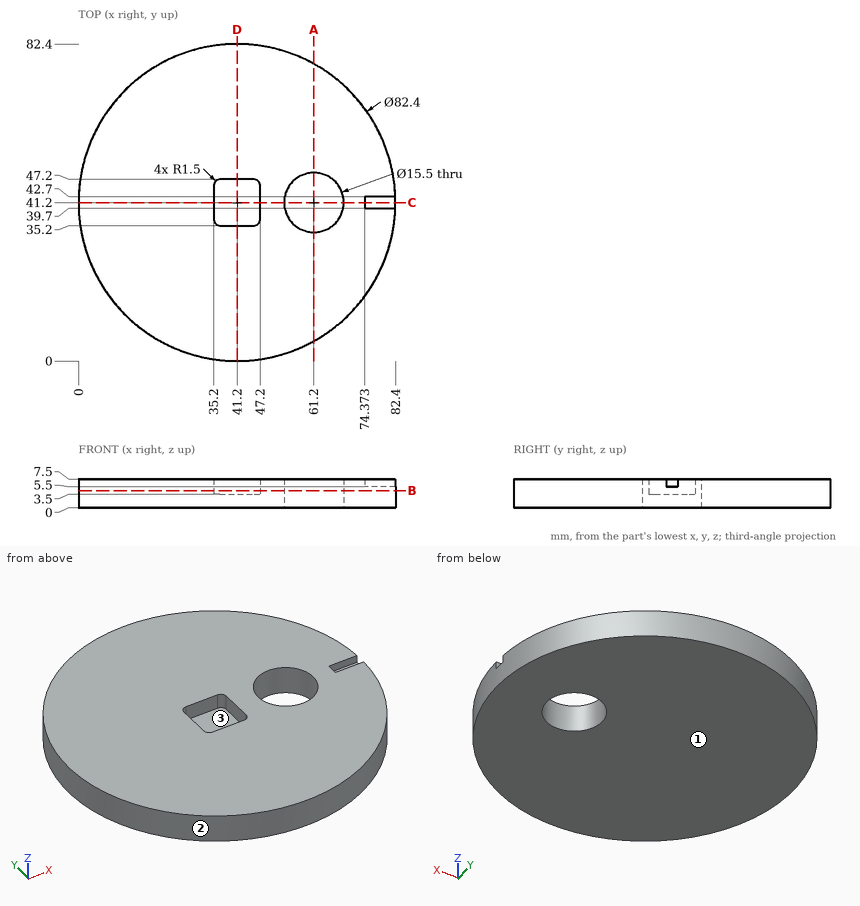
Geometry: see drawing. Coordinates: mm, zero at the bounding-box minimum. Round coordinates to 2 decimals unless told otherwise and drop trailing zeros. Order: outer loops, then holes, each group sorted by start corner. A loop starts at its lowest first (then second) coordinate and runs counter-clockwise, first axis right, second up. Notation, with made-up numbers: (28.5, -22.75) - (57.5, -22.75) arc R19 ccw to (57.5, -2.75) - close; hole circle Ø10 at (23, 33). An arc over 180 degrees is marked (long way). One line per question, with ' | ' between items. Start each with the question number.
1) Cut plane B-B, the plane z = 4.5. Return the cut outline in (x, y).
2) Ray query, probe 1 along X at (y, z) = (41.2, 4.75); probe 2 along X at (y, z) = (41.2, 2); probe 3 along Y at (x, z) = (61.2, 4.5). Return the intervals inside material, ascending.
3) Cut plane C-C, the plane y = 41.2. Return the cut outline in (x, z), then the cut area to 3 significant figures.
4) Cut plane D-D, the plane x = 41.2. Return the cut outline in (y, z).
5) Pull-direction query (X, two-part tool) for the marked faces 1, 2 and 3; classes: +X half, -X half, draft (parallel to the pull), parting line (faces both ways), or undercut.
6) Cut plane A-A, the plane x = 61.2. Return the cut outline in (y, z), then the cut area to 3 significant figures.
7) Contact query for flat-ended pins moving along their axis: P1, Ø4, axis at x = 66, z = 6, coming from the -Y side; P2, Ø0.6, axis at x = 78, z = 6, coming from the +Y side; P3, Ø1.5, axis at x = 44, z = 3, coming from the -Y side. Output: stop coordinate, or through.
Worked out:
1) outline: circle Ø82.4 at (41.2, 41.2); hole (35.2, 36.7) arc R1.5 ccw to (36.7, 35.2) - (45.7, 35.2) arc R1.5 ccw to (47.2, 36.7) - (47.2, 45.7) arc R1.5 ccw to (45.7, 47.2) - (36.7, 47.2) arc R1.5 ccw to (35.2, 45.7) - close; hole circle Ø15.5 at (61.2, 41.2)
2) probe 1: x = 0 to 35.2, 47.2 to 53.45, 68.95 to 82.4 | probe 2: x = 0 to 53.45, 68.95 to 82.4 | probe 3: y = 5.18 to 33.45, 48.95 to 77.22
3) outline: (0, 0) - (53.45, 0) - (53.45, 7.5) - (47.2, 7.5) - (47.2, 3.5) - (35.2, 3.5) - (35.2, 7.5) - (0, 7.5) - close; (68.95, 0) - (82.4, 0) - (82.4, 5.5) - (74.37, 5.5) - (74.37, 7.5) - (68.95, 7.5) - close | area: 438 mm^2
4) outline: (0, 0) - (82.4, 0) - (82.4, 7.5) - (47.2, 7.5) - (47.2, 3.5) - (35.2, 3.5) - (35.2, 7.5) - (0, 7.5) - close
5) face 1: draft | face 2: parting line | face 3: undercut
6) outline: (5.18, 0) - (33.45, 0) - (33.45, 7.5) - (5.18, 7.5) - close; (48.95, 0) - (77.22, 0) - (77.22, 7.5) - (48.95, 7.5) - close | area: 424 mm^2
7) P1: stops at y = 6.88 | P2: stops at y = 60.31 | P3: stops at y = 0.05
